Build history of the part. All positions in model axes, mm. Face numbers are marked on the shaded views. A direction names the side the tool comes from. Round coordinates to 2 decimals unless told otherwise and drop trailing zeros. Write each loop counter-clockwise with the first axis right and the second up, starting at its lowest first coordinate (ties: lowest second). Pieces come first, ordered by that corner, then holes.
1) Saw through at D-D (x = -32). Write the cut outline in (y, z), plus the area to 3 significant figures.
2) Which spindle directions (+Z, -Z, +X, -X, +Y, -Y) get a long thin tool onto all of the face, cutting with end or side? Do the marked faces 1 and 2. Say none if no direction does.
3) Wall check: probe 1 along Y at (x, z) = (-42, -94.5); probe 2 along Z at (x, y) = (-53, 5.5). Give the ranges that are in metal, low to high.
4) Flat gauge pins, fed straight in: pin 1 (12 mm diameter, centred on y = 1, z = -73, fed in from +X); pin 2 (4 mm diameter, centred on x = -34.5, z = -67.5, fed in from -Y); pin 3 (3 mm diameter, centred on x = -46, y = 0.5, fed in from -Z). Where does each tip first touch, or does it go through?
5) Saw through at B-B (y = 14.5). Write the cut outline in (x, z), plus the area to 3 significant figures.
6) Saw through at A-A (x = -53). Write the cut outline in (y, z), plus the area to 3 significant figures.
7) Saw through at C-C (z = -86). Write the cut outline in (x, y).
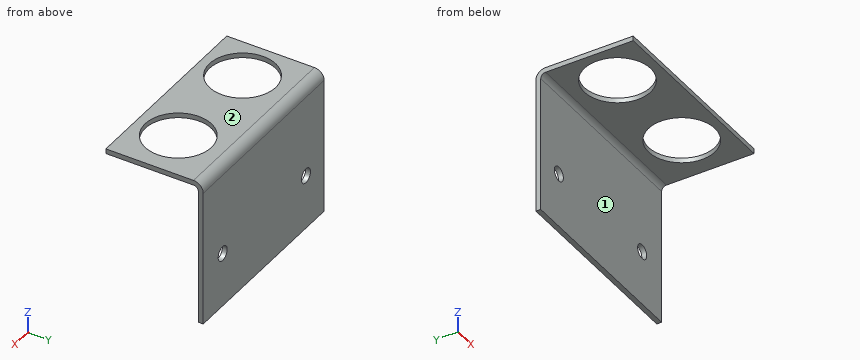
from build123d import *

# Parameters (mm, degrees)
BOSS_EXTRUDE1_DEPTH    = 50.8
SKETCH2_R              = 8.636
CUT_EXTRUDE1_DEPTH     = 88.642940525
CONVERT_SOLID1_START   = -75.861380996
CONVERT_SOLID1_DEPTH   = 50.8
CONVERT_SOLID1_2_DEPTH = 50.8
SKETCH7_R              = 1.89865
CUT_EXTRUDE2_DEPTH     = 129.109840672


# Read off the part's stored shape, not the designer's step: Convert-Solid1
with BuildPart() as part:
    # Sketch1 → Boss-Extrude1 (new body)
    with BuildSketch(Plane(origin=(-25.061380996, 0, 0), x_dir=(0, 0, -1), z_dir=(1, 0, 0))):
        Polygon((63.543927145, -3.611794537), (63.543927145, 20.518205463), (100.373927145, 20.518205463), (100.373927145, 21.788205463), (62.273927145, 21.788205463), (62.273927145, -3.611794537), align=None)
    extrude(amount=-BOSS_EXTRUDE1_DEPTH)

    # Sketch2 → Cut-Extrude1 (cut, through all)
    with BuildSketch(Plane.XY.offset(-62.273927145)):
        with Locations((-64.852637296, 7.338590118)):
            Circle(SKETCH2_R)
        with Locations((-37.852637296, 7.338590118)):
            Circle(SKETCH2_R)
    extrude(amount=-CUT_EXTRUDE1_DEPTH, mode=Mode.SUBTRACT)

    # Convert-Solid1 outline → Convert-Solid1 (cut)
    with BuildSketch(Plane.YZ.offset(CONVERT_SOLID1_START)):
        with BuildLine():
            Line((21.788205463, -62.273927145), (19.248205463, -62.273927145))
            ThreePointArc((19.248205463, -62.273927145), (21.044256687, -63.01787592), (21.788205463, -64.813927145))
            Line((21.788205463, -64.813927145), (21.788205463, -62.273927145))
        make_face()
    extrude(amount=CONVERT_SOLID1_DEPTH, mode=Mode.SUBTRACT)

    # Convert-Solid1 2 outline → Convert-Solid1 2 (add)
    with BuildSketch(Plane.YZ.offset(CONVERT_SOLID1_START)):
        with BuildLine():
            Line((20.518205463, -63.543927145), (19.248205463, -63.543927145))
            ThreePointArc((19.248205463, -63.543927145), (20.146231075, -63.915901533), (20.518205463, -64.813927145))
            Line((20.518205463, -64.813927145), (20.518205463, -63.543927145))
        make_face()
    extrude(amount=CONVERT_SOLID1_2_DEPTH)

    # Sketch7 → Cut-Extrude2 (cut, through all)
    with BuildSketch(Plane(origin=(0, 20.518205463, 0), x_dir=(-1, 0, 0), z_dir=(0, -1, 0))):
        with Locations(Location((68.241380996, 86.126775189, 0), (0, 0, 90))):
            Circle(SKETCH7_R)
        with Locations(Location((33.236646392, 86.126775189, 0), (0, 0, 90))):
            Circle(SKETCH7_R)
    extrude(amount=-CUT_EXTRUDE2_DEPTH, mode=Mode.SUBTRACT)


solid = part.part
Evaluation:
1. outline: (-3.61, -63.54) - (0.99, -63.54) - (0.99, -62.27) - (-3.61, -62.27) - close; (13.69, -63.54) - (19.25, -63.54) arc R1.27 cw to (20.52, -64.81) - (20.52, -84.69) - (21.79, -84.69) - (21.79, -64.81) arc R2.54 ccw to (19.25, -62.27) - (13.69, -62.27) - close; (20.52, -100.37) - (21.79, -100.37) - (21.79, -87.57) - (20.52, -87.57) - close
1. area: 58.2 mm2
2. face 1: -Z, +X, -X, -Y
2. face 2: +Z, +X, -X, +Y, -Y
3. probe 1: y = 20.52 to 21.79
3. probe 2: z = -63.54 to -62.27
4. pin 1: passes through
4. pin 2: stops at y = 20.52
4. pin 3: stops at z = -63.54
5. outline: (-75.86, -63.54) - (-69.68, -63.54) - (-69.68, -62.27) - (-75.86, -62.27) - close; (-60.03, -63.54) - (-42.68, -63.54) - (-42.68, -62.27) - (-60.03, -62.27) - close; (-33.03, -63.54) - (-25.06, -63.54) - (-25.06, -62.27) - (-33.03, -62.27) - close
5. area: 40.0 mm2
6. outline: (-3.61, -63.54) - (19.25, -63.54) arc R1.27 cw to (20.52, -64.81) - (20.52, -100.37) - (21.79, -100.37) - (21.79, -64.81) arc R2.54 ccw to (19.25, -62.27) - (-3.61, -62.27) - close
6. area: 78.0 mm2
7. outline: (-75.86, 20.52) - (-70.14, 20.52) - (-70.14, 21.79) - (-75.86, 21.79) - close; (-66.35, 20.52) - (-35.13, 20.52) - (-35.13, 21.79) - (-66.35, 21.79) - close; (-31.34, 20.52) - (-25.06, 20.52) - (-25.06, 21.79) - (-31.34, 21.79) - close
